from build123d import *

# Parameters (mm, degrees)
F1_DEPTH  = 12.7
F3_DEPTH  = 82.55
F7_R      = 2.2225
F8_DEPTH  = 107.951
F10_DEPTH = 9.525


with BuildPart() as f1:
    # F0 (on Top) → F1 (new body)
    with BuildSketch(Plane.XY):
        with BuildLine():
            Line((13.9777885884, 5.014068319), (-9.1354904962, 8.7746195582))
            ThreePointArc((-9.1354904962, 8.7746195582), (-19.453128969, 0), (-9.1354904962, -8.7746195582))
            Line((-9.1354904962, -8.7746195582), (13.9777885884, -5.014068319))
            ThreePointArc((13.9777885884, -5.014068319), (18.2419951753, 0), (13.9777885884, 5.014068319))
        make_face()
    extrude(amount=F1_DEPTH)

    # F2 (on face) → F3 (join)
    with BuildSketch(Plane.XY.offset(12.7)):
        with BuildLine():
            Line((-9.293128969, 8.89), (-10.563128969, 8.89))
            ThreePointArc((-10.563128969, 8.89), (-19.453128969, 0), (-10.563128969, -8.89))
            Line((-10.563128969, -8.89), (-9.293128969, -8.89))
            ThreePointArc((-9.293128969, -8.89), (-0.403128969, 0), (-9.293128969, 8.89))
        make_face()
    extrude(amount=F3_DEPTH)

    # F5 (on Front) → F6 (revolve)
    with BuildSketch(Plane.XZ):
        Polygon((-13.484128969, 95.25), (-7.705628969, 95.25), (-8.023128969, 107.95), (-13.484128969, 107.95), align=None)
    revolve(axis=Axis((-13.484128969, 0, 63.5), (0, 0, 1)))

    # F7 (on face) → F8 (cut, through all)
    with BuildSketch(Plane.XY.offset(107.95)):
        with Locations((-13.484128969, 0)):
            Circle(F7_R)
    extrude(amount=-F8_DEPTH, mode=Mode.SUBTRACT)

    # F9 (on face) → F10 (cut)
    with BuildSketch(Plane.XY.offset(12.7)):
        with BuildLine():
            Line((13.5698918818, 2.5070341595), (1.2057433852, 4.5186922103))
            ThreePointArc((1.2057433852, 4.5186922103), (2.136871031, 0), (1.2057433852, -4.5186922103))
            Line((1.2057433852, -4.5186922103), (13.5698918818, -2.5070341595))
            ThreePointArc((13.5698918818, -2.5070341595), (15.7019951753, 0), (13.5698918818, 2.5070341595))
        make_face()
    extrude(amount=-F10_DEPTH, mode=Mode.SUBTRACT)


solid = f1.part
Can you work these out from the model? Positions are in its coordinate system, mm. A direction names the side the tool comes from. Coordinates: 2 decimals unless noted, no trailing zeros. Order: outer loops, then holes, each group sorted by start corner. A loop starts at its lowest first (then second) coordinate and runs counter-clockwise, first axis right, second up. Notation, with made-up numbers: (83, -16.75) -> (135, -16.75) arc R13 cw to (135, 5.25) -> close; hole circle Ø2 at (75, 9.25). An arc over 180 degrees is marked (long way). Use one line per item in the form item = value.
Q1. Imagine slicing it at B-B, the plane z = 63. List the corners of the cut face in (x, y) for me (1 decimal).
From the geometry:
outline = (-10.6, -8.9) -> (-9.3, -8.9) arc R8.9 ccw to (-9.3, 8.9) -> (-10.6, 8.9) arc R8.9 ccw to start; hole circle Ø4.4 at (-13.5, 0)
Q2. Which directions (+Z, -Z, +X, -X, +Y, -Y) give clear straight access to the entire face, cutting with the end or side of a thin tool? Please do faces 1 (the face through (-13.6, -2.4, 107.95)), 2 (the face through (-0.405, -0.195, 53.397)), 3 (the face through (8, 0, 3.175)).
From the geometry:
face_1 = +Z, +X, -X, +Y, -Y
face_2 = +Z, +X
face_3 = +Z
Q3. Imagine slicing it at D-D, the plane z = 97. List the corners of the cut face in (x, y) for me (1 decimal), then the cut area to 3 significant figures.
From the geometry:
outline = circle Ø11.5 at (-13.5, 0); hole circle Ø4.4 at (-13.5, 0)
area = 87.8 mm²
Q4. Will these pins go through, and if not, where does the flat tip stop? P1, Ø7, axis at x = 9.5, y = -1, coming from the +Z side; P2, Ø8, axis at x = -5, z = 62, coming from the -Y side; P3, Ø5, axis at y = -5, z = 33.5, coming from the +X side; P4, Ø2.5, axis at x = -13.48, y = 0, coming from the +Z side.
From the geometry:
P1 = 12.7
P2 = -8.89
P3 = -0.76
P4 = through
Q5. Imagine slicing it at C-C, the plane x = 8. List the corners of the cut face in (y, z) for me (3 decimals).
From the geometry:
outline = (-5.987, 0) -> (5.987, 0) -> (5.987, 12.7) -> (3.413, 12.7) -> (3.413, 3.175) -> (-3.413, 3.175) -> (-3.413, 12.7) -> (-5.987, 12.7) -> close
Q6. I need wall thicknesses on L1, parallel to X at y = -0.25, z = 67; L2, parallel to Z at x = -1.5, y = 5.75; L3, parallel to Z at x = -3, y = 2.75. Which ranges of each line are inside material? Lowest first, please.
From the geometry:
L1 = -19.45 to -15.69, -11.28 to -0.41
L2 = 0 to 12.7
L3 = 0 to 95.25
Q7. Imagine slicing it at A-A, the plane y = 0. List the corners of the cut face in (x, z) for me (3 decimals), then the cut area to 4 significant figures.
From the geometry:
outline = (-19.453, 0) -> (-15.707, 0) -> (-15.707, 107.95) -> (-18.945, 107.95) -> (-19.263, 95.25) -> (-19.453, 95.25) -> close; (-11.262, 0) -> (18.242, 0) -> (18.242, 12.7) -> (15.702, 12.7) -> (15.702, 3.175) -> (2.137, 3.175) -> (2.137, 12.7) -> (-0.403, 12.7) -> (-0.403, 95.25) -> (-7.706, 95.25) -> (-8.023, 107.95) -> (-11.262, 107.95) -> close
area = 1,585 mm²
Q8. We'd pull the mould along Y, two halves only. Please class faces 4 (the face through (7.47, 3.5, 8)), 5 (the face through (2.58, 6.87, 6.26)), 6 (the face through (2.137, 0.065, 8.004)), 7 (the face through (-1, 0, 0)): released by +Y, released by -Y, zero draft, split by the parting line, or undercut.
From the geometry:
face_4 = undercut
face_5 = released by +Y
face_6 = undercut
face_7 = zero draft
